from build123d import *

# Parameters (mm, degrees)
BOSS_EXTRUDE1_DEPTH = 7
BOSS_EXTRUDE3_DEPTH = 10
SKETCH6_R           = 1.35
CUT_EXTRUDE3_DEPTH  = 8.5


with BuildPart() as part:
    # Sketch1 → Boss-Extrude1 (new body)
    with BuildSketch(Plane.XY):
        with BuildLine():
            ThreePointArc((5.050452833, -4.633288902), (-0.057176836, -7.835700867), (-5.249547167, -4.77259565))
            Line((-5.249547167, -4.77259565), (-5.135937781, -13.17259565))
            Line((-5.135937781, -13.17259565), (5.164062219, -13.033288902))
            Line((5.164062219, -13.033288902), (5.050452833, -4.633288902))
        make_face()
        with BuildLine():
            ThreePointArc((5.664385761, -2.036231273), (-1.546144107, 3.589638037), (-5.249547167, -4.77259565))
            Line((-5.249547167, -4.77259565), (5.050452833, -4.633288902))
            ThreePointArc((5.050452833, -4.633288902), (5.508816158, -3.370549635), (5.664385761, -2.036231273))
        make_face()
        with BuildLine():
            Line((5.050452833, -4.633288902), (-5.249547167, -4.77259565))
            ThreePointArc((-5.249547167, -4.77259565), (-0.057176836, -7.835700867), (5.050452833, -4.633288902))
        make_face()
    extrude(amount=BOSS_EXTRUDE1_DEPTH)

    # Sketch2 → Boss-Extrude3 (add)
    with BuildSketch(Plane.XY.offset(7)):
        with BuildLine():
            Line((5.063146119, -5.571799449), (5.912597424, -5.560310683))
            ThreePointArc((5.912597424, -5.560310683), (6.622250869, -3.861405013), (6.864385761, -2.036231273))
            ThreePointArc((6.864385761, -2.036231273), (-2.052012342, 4.696332749), (-6.086305185, -5.722594964))
            Line((-6.086305185, -5.722594964), (-5.236853881, -5.711106197))
            Line((-5.236853881, -5.711106197), (-5.249547167, -4.77259565))
            ThreePointArc((-5.249547167, -4.77259565), (-0.214051642, 3.763238321), (5.050452833, -4.633288902))
            Line((5.050452833, -4.633288902), (5.063146119, -5.571799449))
        make_face()
        with BuildLine():
            Line((1.811820806, -5.615773387), (5.063146119, -5.571799449))
            Line((5.063146119, -5.571799449), (5.050452833, -4.633288902))
            ThreePointArc((5.050452833, -4.633288902), (-0.214051642, 3.763238321), (-5.249547167, -4.77259565))
            Line((-5.249547167, -4.77259565), (-5.236853881, -5.711106197))
            Line((-5.236853881, -5.711106197), (-1.985528568, -5.66713226))
            ThreePointArc((-1.985528568, -5.66713226), (-2.264842281, 1.438248968), (3.939385761, -2.036231273))
            ThreePointArc((3.939385761, -2.036231273), (3.367343284, -4.118276805), (1.811820806, -5.615773387))
        make_face()
        with BuildLine():
            Line((5.078495254, -6.706676883), (5.063146119, -5.571799449))
            Line((5.063146119, -5.571799449), (1.811820806, -5.615773387))
            ThreePointArc((1.811820806, -5.615773387), (-0.080505202, -6.110858617), (-1.985528568, -5.66713226))
            Line((-1.985528568, -5.66713226), (-5.236853881, -5.711106197))
            Line((-5.236853881, -5.711106197), (-5.221504746, -6.845983631))
            ThreePointArc((-5.221504746, -6.845983631), (-0.040948408, -9.035591128), (5.078495254, -6.706676883))
        make_face()
        with BuildLine():
            Line((5.164062219, -13.033288902), (5.078495254, -6.706676883))
            ThreePointArc((5.078495254, -6.706676883), (-0.040948408, -9.035591128), (-5.221504746, -6.845983631))
            Line((-5.221504746, -6.845983631), (-5.135937781, -13.17259565))
            Line((-5.135937781, -13.17259565), (5.164062219, -13.033288902))
        make_face()
        with BuildLine():
            Line((6.06137162, -16.560310683), (5.912597424, -5.560310683))
            ThreePointArc((5.912597424, -5.560310683), (5.524642674, -6.154664432), (5.078495254, -6.706676883))
            Line((5.078495254, -6.706676883), (5.164062219, -13.033288902))
            Line((5.164062219, -13.033288902), (-5.135937781, -13.17259565))
            Line((-5.135937781, -13.17259565), (-5.221504746, -6.845983631))
            ThreePointArc((-5.221504746, -6.845983631), (-5.6824181, -6.30623911), (-6.086305185, -5.722594964))
            Line((-6.086305185, -5.722594964), (-5.937530989, -16.722594964))
            Line((-5.937530989, -16.722594964), (6.06137162, -16.560310683))
        make_face()
        with BuildLine():
            ThreePointArc((5.078495254, -6.706676883), (5.524642674, -6.154664432), (5.912597424, -5.560310683))
            Line((5.912597424, -5.560310683), (5.063146119, -5.571799449))
            Line((5.063146119, -5.571799449), (5.078495254, -6.706676883))
        make_face()
        with BuildLine():
            Line((-5.236853881, -5.711106197), (-6.086305185, -5.722594964))
            ThreePointArc((-6.086305185, -5.722594964), (-5.6824181, -6.30623911), (-5.221504746, -6.845983631))
            Line((-5.221504746, -6.845983631), (-5.236853881, -5.711106197))
        make_face()
    extrude(amount=BOSS_EXTRUDE3_DEPTH)

    # Sketch6 → Cut-Extrude3 (cut)
    with BuildSketch(Plane(origin=(0.225044595, -16.639246579, 0), x_dir=(-0.999908551, -0.01352369, 0), z_dir=(0.01352369, -0.999908551, 0))):
        with Locations((0.241163233, -13)):
            Circle(SKETCH6_R)
    extrude(amount=-CUT_EXTRUDE3_DEPTH, mode=Mode.SUBTRACT)


solid = part.part
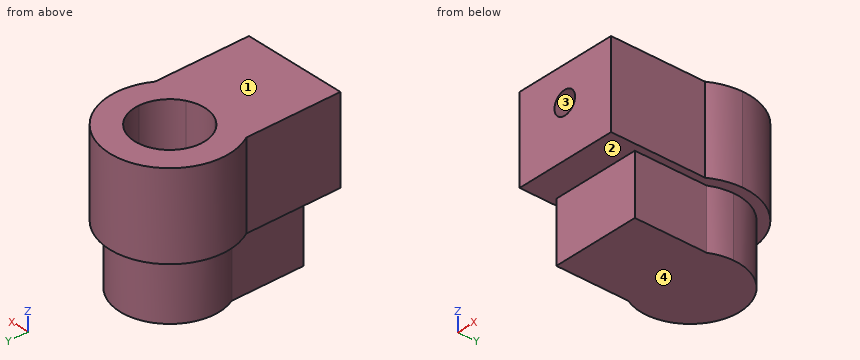
Read the model definition and answer for the solid it produces. Units are mm, in the model's axes. Face numbers are marked on the shaded views. A direction names the side the tool comes from. Give positions to 0.01 mm unless a question says otherwise; leave off trailing zeros. Write each loop counter-clockwise with the first axis right and the second up, starting at its lowest first coordinate (ties: lowest second). Pieces come first, ordered by that corner, then holes. Notation, with made-up numbers: (-36.75, 48.5) -> (-24.75, 48.5) arc R13 cw to (-24.75, 61.5) -> close; hole circle Ø5 at (16, 60.25). An arc over 180 degrees is marked (long way). Answer as a JSON object with one key per item and string values. Group by question number.
1) A tool of negligible diameter and unlimited length cuts with its end or side. For the marked faces 1 and 2, from which of +Z, -Z, +X, -X, +Y, -Y can it reach the whole face along a straight path? Write none if from no direction.
2) Find section C-C (x = -3). Write down the section's boundary in (y, z), and give its area (3 significant figures).
3) Each of these flat-tipped pins is pushed along its axis until it touches: P1, Ø1.5, axis at x = 2, z = 8.5, coming from the -Y side; P2, Ø2, axis at x = -4.5, z = 12.5, coming from the -Y side; P3, Ø5, axis at x = -5.5, z = 8, coming from the +Y side. Where does it stop, or does it pass through?
4) Find section B-B (y = -1.75). Write down the section's boundary in (x, z), and give its area (3 significant figures).
5) Find section D-D (z = 2.5). Write down the section's boundary in (x, y), and give its area (3 significant figures).
6) Consider L1, parallel to X at y = -2, z = 16; L2, parallel to Z at x = -4.75, y = -15.25; L3, parallel to Z at x = -3.25, y = -3.5. Determine where each line is inside the solid, lowest interval first. Write a range as from..to.
7) The mould has two halves that part along X. Classify the marked faces 3 and 4: +X half, -X half, draft (parallel to the pull), parting line (faces both ways), or undercut.
8) Find section A-A (z = 15). Write down the section's boundary in (x, y) (3 decimals).
Values follow:
{
 "1": {"face 1": "+Z, +X, -X, +Y, -Y", "face 2": "-Z"},
 "2": {"outline": "(-16.68, 7) -> (-13.14, 7) -> (-13.14, 0) -> (3.01, 0) -> (3.01, 7) -> (4.35, 7) -> (4.35, 17) -> (0.86, 17) -> (0.86, 7) -> (-4.93, 7) -> (-4.93, 17) -> (-16.68, 17) -> close", "area": "265 mm2"},
 "3": {"P1": "stops at y = -16.63", "P2": "stops at y = -16.72", "P3": "stops at y = 4.35"},
 "4": {"outline": "(-7.13, 7) -> (-5.93, 7) -> (-5.93, 0) -> (5.66, 0) -> (5.66, 7) -> (6.86, 7) -> (6.86, 17) -> (3.93, 17) -> (3.93, 7) -> (-4.2, 7) -> (-4.2, 17) -> (-7.13, 17) -> close", "area": "140 mm2"},
 "5": {"outline": "(-5.25, -4.77) -> (-5.14, -13.17) -> (5.16, -13.03) -> (5.05, -4.63) arc R5.8 ccw (long way) to start", "area": "169 mm2"},
 "6": {"L1": "x = -7.14..-4.21, 3.94..6.86", "L2": "z = 7..17", "L3": "z = 0..7"},
 "7": {"face 3": "undercut", "face 4": "draft"},
 "8": {"outline": "(-6.086, -5.723) -> (-5.938, -16.723) -> (6.061, -16.56) -> (5.913, -5.56) arc R7 ccw (long way) to start; hole circle Ø8.15 at (-0.136, -2.036)"}
}
